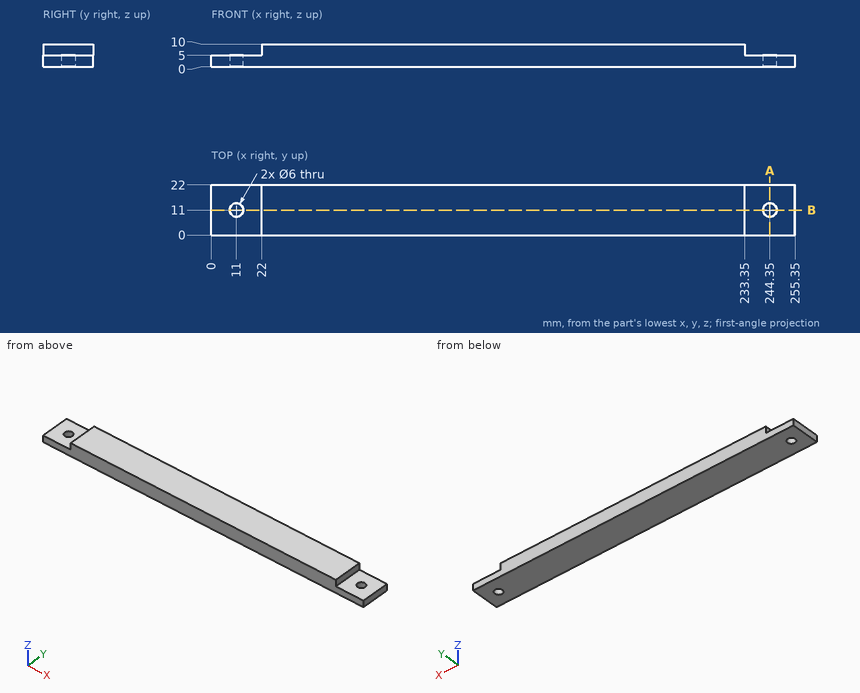
The drawing under review shows one solid part. Ordinate dimensions are in mm from its lowest x, y, z. Coordinates: 2 decimals unless noted, no trailing zeros. Order: outer loops, then holes, each group sorted by start corner. A loop starts at its lowest first (then second) coordinate and runs counter-clockwise, first axis right, second up. Notation, with made-up numbers: (64, 1.25) -> (101, 1.25) arc R15 ccw to (101, 27.25) -> close; hole circle Ø6 at (66, 78.5). An arc over 180 degrees is marked (long way). Return JSON: item names as keys, results as strings.
1. For line 1 (X direction, y = 11, z = 3.05); line 2 (Y direction, x = 244.35, z = 2.55); line 3 (X direction, y = 9.75, z = 1), list the stretches that pass through material, from the lowest coordinate up. Write a range as from..to.
Answer block:
{"line 1": "0..8, 14..241.35, 247.35..255.35", "line 2": "0..8, 14..22", "line 3": "0..8.27, 13.73..241.62, 247.08..255.35"}
2. We need section B-B on y = 11. Write out the cut boundary in (x, z).
Answer block:
{"outline": "(0, 0) -> (8, 0) -> (8, 5) -> (0, 5) -> close; (14, 0) -> (241.35, 0) -> (241.35, 5) -> (233.35, 5) -> (233.35, 10) -> (22, 10) -> (22, 5) -> (14, 5) -> close; (247.35, 0) -> (255.35, 0) -> (255.35, 5) -> (247.35, 5) -> close"}
3. For pin 1 Ø11 at (x, y) = (9, 8) entering from +Z; pin 2 Ø1 at (y, z) = (13, 9) entering from -X; pin 3 Ø1.5 at (y, z) = (4.5, 7.5) entering from +X, all flat-tipped, find the tip position at first contact; note any pin that passes through.
Answer block:
{"pin 1": "z = 5", "pin 2": "x = 22", "pin 3": "x = 233.35"}
4. We need section A-A on x = 244.35. Write out the cut boundary in (y, z), and give its area (3 significant figures).
Answer block:
{"outline": "(0, 0) -> (8, 0) -> (8, 5) -> (0, 5) -> close; (14, 0) -> (22, 0) -> (22, 5) -> (14, 5) -> close", "area": "80.0 mm²"}
